```python
from build123d import *

# Parameters (mm, degrees)
ESBO_O1_W                = 6
ESBO_O1_H                = 6
RESSALTO_EXTRUS_O1_DEPTH = 3.4
ESBO_O2_R                = 1.75
RESSALTO_EXTRUS_O2_DEPTH = 1.6
ESBO_O3_R                = 0.75
RESSALTO_EXTRUS_O3_DEPTH = 0.5
ESBO_O5_W                = 0.3
ESBO_O5_H                = 0.5
RESSALTO_EXTRUS_O4_DEPTH = 4.27
ESBO_O6_W                = 6
ESBO_O6_H                = 6
CORTE_EXTRUS_O1_DEPTH    = 0.6
ESBO_O7_W                = 6
ESBO_O7_H                = 6
RESSALTO_EXTRUS_O5_DEPTH = 0.6
ESBO_O9_W                = 6
ESBO_O9_H                = 6
CORTE_EXTRUS_O2_DEPTH    = 0.2
ESBO_O10_W               = 5.8
ESBO_O10_H               = 5.8
RESSALTO_EXTRUS_O6_DEPTH = 0.1
FILETE3_R                = 0.5
FILETE4_R                = 0.5
ESBO_O12_R               = 1.75
ESBO_O12_R_2             = 0.759056116
ESBO_O12_R_3             = 0.75
RESSALTO_EXTRUS_O7_DEPTH = 0.5


with BuildPart() as part:
    # Esboço1 → Ressalto-extrusão1 (new body)
    with BuildSketch(Plane(origin=(0, 0, 0), x_dir=(1, 0, 0), z_dir=(0, 1, 0))):
        with Locations((-7, 7.272727273)):
            Rectangle(ESBO_O1_W, ESBO_O1_H)
    extrude(amount=RESSALTO_EXTRUS_O1_DEPTH)

    # Esboço2 → Ressalto-extrusão2 (add)
    with BuildSketch(Plane(origin=(0, 3.4, 0), x_dir=(1, 0, 0), z_dir=(0, 1, 0))):
        with Locations((-7, 7.272727273)):
            Circle(ESBO_O2_R)
    extrude(amount=RESSALTO_EXTRUS_O2_DEPTH)

    # Esboço3 → Ressalto-extrusão3 (add)
    with BuildSketch(Plane(origin=(0, 3.4, 0), x_dir=(1, 0, 0), z_dir=(0, 1, 0))):
        with Locations((-9, 9.272727273)):
            Circle(ESBO_O3_R)
        with Locations((-5, 9.272727273)):
            Circle(ESBO_O3_R)
        with Locations((-9, 5.272727273)):
            Circle(ESBO_O3_R)
        with Locations((-5, 5.272727273)):
            Circle(ESBO_O3_R)
    extrude(amount=RESSALTO_EXTRUS_O3_DEPTH)

    # Esboço5 → Ressalto-extrusão4 (add)
    with BuildSketch(Plane.XZ):
        with Locations((-9.5, -7.272727273)):
            Rectangle(ESBO_O5_W, ESBO_O5_H)
        with Locations((-4.452085856, -7.272727273)):
            Rectangle(ESBO_O5_W, ESBO_O5_H)
    extrude(amount=RESSALTO_EXTRUS_O4_DEPTH)

    # Esboço6 → Corte-extrusão1 (cut)
    with BuildSketch(Plane(origin=(0, 3.4, 0), x_dir=(1, 0, 0), z_dir=(0, 1, 0))):
        with Locations((-7, 7.272727273)):
            Rectangle(ESBO_O6_W, ESBO_O6_H)
    extrude(amount=-CORTE_EXTRUS_O1_DEPTH, mode=Mode.SUBTRACT)

    # Esboço7 → Ressalto-extrusão5 (add)
    with BuildSketch(Plane(origin=(0, 2.8, 0), x_dir=(1, 0, 0), z_dir=(0, 1, 0))):
        with Locations((-7, 7.272727273)):
            Rectangle(ESBO_O7_W, ESBO_O7_H)
    extrude(amount=RESSALTO_EXTRUS_O5_DEPTH)

    # Esboço9 → Corte-extrusão2 (cut)
    with BuildSketch(Plane(origin=(0, 3.4, 0), x_dir=(1, 0, 0), z_dir=(0, 1, 0))):
        with Locations((-7, 7.272727273)):
            Rectangle(ESBO_O9_W, ESBO_O9_H)
    extrude(amount=-CORTE_EXTRUS_O2_DEPTH, mode=Mode.SUBTRACT)

    # Esboço10 → Ressalto-extrusão6 (add)
    with BuildSketch(Plane(origin=(0, 3.2, 0), x_dir=(1, 0, 0), z_dir=(0, 1, 0))):
        with Locations((-7, 7.272727273)):
            Rectangle(ESBO_O10_W, ESBO_O10_H)
    extrude(amount=RESSALTO_EXTRUS_O6_DEPTH)

    # Filete3
    filete3_edges = [part.edges().sort_by_distance(p)[0] for p in [
        (-9.9, 3.25, -10.172727273),
        (-9.9, 3.25, -4.372727273),
        (-4.1, 3.25, -4.372727273),
        (-4.1, 3.25, -10.172727273),
    ]]
    fillet(filete3_edges, radius=FILETE3_R)

    # Filete4
    filete4_edges = [part.edges().sort_by_distance(p)[0] for p in [
        (-10, 1.6, -10.272727273),
        (-10, 1.6, -4.272727273),
        (-4, 1.6, -4.272727273),
        (-4, 1.6, -10.272727273),
    ]]
    fillet(filete4_edges, radius=FILETE4_R)

    # Esboço12 → Ressalto-extrusão7 (add)
    with BuildSketch(Plane(origin=(0, 3.3, 0), x_dir=(1, 0, 0), z_dir=(0, 1, 0))):
        with Locations((-7, 7.272727273)):
            Circle(ESBO_O12_R)
        with Locations((-9, 9.272727273)):
            Circle(ESBO_O12_R_2)
        with Locations((-5, 9.272727273)):
            Circle(ESBO_O12_R_3)
        with Locations((-5, 5.272727273)):
            Circle(ESBO_O12_R_3)
        with Locations((-9, 5.272727273)):
            Circle(ESBO_O12_R_3)
    extrude(amount=RESSALTO_EXTRUS_O7_DEPTH)


solid = part.part
```
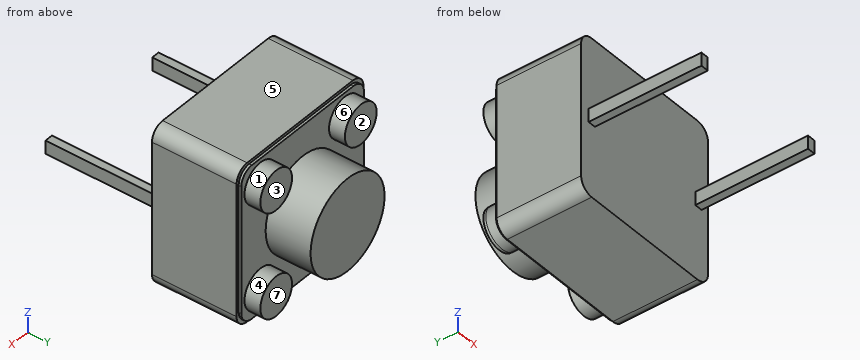
Design review of the part built by this model. Coordinates are the model's own, in mm. Face numbers are marked on the shaded views. A direction names the side the tool comes from. Give positions to 0.01 mm unless a question says otherwise; leave off trailing zeros. Write each loop counter-clockwise with the first axis right and the second up, starting at its lowest first coordinate (ties: lowest second). Pieces come first, ordered by that corner, then holes.
(1) Add section A-A (x = -7). Give the boundary of the cut face in (y, z).
Checked values:
outline: (0, -10.27) - (3.2, -10.27) - (3.2, -10.17) - (3.3, -10.17) - (3.3, -9.02) - (5, -9.02) - (5, -5.52) - (3.3, -5.52) - (3.3, -4.37) - (3.2, -4.37) - (3.2, -4.27) - (0, -4.27) - close
(2) Clearance check with flat-ended pins moving along their axes: pin 1 Ø3 at (x, z) = (-7.5, -7) entering from -Y; pin 2 Ø1.6 at (x, z) = (-9, -9) entering from +Y. State where each tip first meets the part, or that it passes through.
Checked values:
pin 1: stops at y = 0
pin 2: stops at y = 3.9
(3) Add section D-D (x = -5). Give the boundary of the cut face in (y, z).
Checked values:
outline: (0, -10.27) - (3.2, -10.27) - (3.2, -10.17) - (3.3, -10.17) - (3.3, -10.02) - (3.9, -10.02) - (3.9, -8.52) - (3.3, -8.52) - (3.3, -6.02) - (3.9, -6.02) - (3.9, -4.52) - (3.3, -4.52) - (3.3, -4.37) - (3.2, -4.37) - (3.2, -4.27) - (0, -4.27) - close
(4) Add section C-C (y = 3.5). Give the boundary of the cut face in (x, z), and give its area (3 significant figures).
Checked values:
outline: circle Ø1.52 at (-9, -9.27); circle Ø1.5 at (-9, -5.27); circle Ø3.5 at (-7, -7.27); circle Ø1.5 at (-5, -9.27); circle Ø1.5 at (-5, -5.27)
area: 16.7 mm2
(5) Mouldability with a two-part tool opening along Z and no side actions: class the marked faces 4, 5, 6 and 7 as +Z half, -Z half, draft (parallel to the pull), parting line (faces both ways), or undercut.
Checked values:
face 4: undercut
face 5: +Z half
face 6: undercut
face 7: draft
(6) Wall thickness on line 1 along Y through (x, z) = (-6.4, -5.5); line 2 along Y through (x, z) = (-6.25, -8.75); line 3 along Z through (x, y) = (-9.4, -0.75): over which ranges is each line inside the solid? List them lowest first.
Checked values:
line 1: y = 0 to 3.3
line 2: y = 0 to 5
line 3: z = -7.52 to -7.02
(7) Tool access review of the marked faces 1, 2 and 3: name each direction out of +Z, -Z, +X, -X, +Y, -Y from which nothing blocks a thin tool from reaching the whole face with its end or side.
Checked values:
face 1: +Y
face 2: +Z, -X, +Y
face 3: +Z, +X, +Y
